from build123d import *

# Parameters (mm, degrees)
SKETCH1_W           = 24
SKETCH1_H           = 24
BOSS_EXTRUDE1_DEPTH = 40
SHELL3_T            = -2
SKETCH3_R           = 11.1
BOSS_EXTRUDE3_DEPTH = 15
SKETCH4_R           = 9.55
CUT_EXTRUDE3_DEPTH  = 12
FILLET4_R           = 0.5
SKETCH2_W           = 20
SKETCH2_H           = 2
BOSS_EXTRUDE5_DEPTH = 40
SKETCH6_W           = 20
SKETCH6_H           = 4
CUT_EXTRUDE4_DEPTH  = 8
SKETCH7_W           = 4
SKETCH7_H           = 18
CUT_EXTRUDE5_DEPTH  = 8
SKETCH8_R           = 2.5
CUT_EXTRUDE6_DEPTH  = 2


with BuildPart() as part:
    # Sketch1 → Boss-Extrude1 (new body)
    with BuildSketch(Plane(origin=(0, 0, 0), x_dir=(1, 0, 0), z_dir=(0, 1, 0))):
        Rectangle(SKETCH1_W, SKETCH1_H)
    extrude(amount=BOSS_EXTRUDE1_DEPTH)

    # Shell3
    shell3_openings = [part.faces().sort_by_distance(p)[0] for p in [
        (0, 40, 0),
        (0, 0, 0),
    ]]
    offset(amount=SHELL3_T, openings=shell3_openings, kind=Kind.INTERSECTION)

    # Sketch3 → Boss-Extrude3 (add)
    with BuildSketch(Plane.XY.offset(12)):
        with Locations((0, 20)):
            Circle(SKETCH3_R)
    extrude(amount=BOSS_EXTRUDE3_DEPTH)

    # Sketch4 → Cut-Extrude3 (cut)
    with BuildSketch(Plane.XY.offset(27)):
        with Locations((0, 20)):
            Circle(SKETCH4_R)
    extrude(amount=-CUT_EXTRUDE3_DEPTH, mode=Mode.SUBTRACT)

    # Fillet4
    fillet4_edges = [part.edges().sort_by_distance(p)[0] for p in [
        (-11.1, 20, 12),
    ]]
    fillet(fillet4_edges, radius=FILLET4_R)

    # Sketch2 → Boss-Extrude5 (add)
    with BuildSketch(Plane(origin=(0, 40, 0), x_dir=(1, 0, 0), z_dir=(0, 1, 0))):
        with Locations((0, 1)):
            Rectangle(SKETCH2_W, SKETCH2_H)
    extrude(amount=-BOSS_EXTRUDE5_DEPTH)

    # Sketch6 → Cut-Extrude4 (cut)
    with BuildSketch(Plane(origin=(11.1, 0, 0), x_dir=(0, 0, -1), z_dir=(1, 0, 0))):
        with Locations((-27, 20)):
            Rectangle(SKETCH6_W, SKETCH6_H)
    extrude(amount=-CUT_EXTRUDE4_DEPTH, mode=Mode.SUBTRACT)

    # Sketch7 → Cut-Extrude5 (cut)
    with BuildSketch(Plane(origin=(0, 8.9, 0), x_dir=(1, 0, 0), z_dir=(0, 1, 0))):
        with Locations((0, -27)):
            Rectangle(SKETCH7_W, SKETCH7_H)
    extrude(amount=CUT_EXTRUDE5_DEPTH, mode=Mode.SUBTRACT)

    # Sketch8 → Cut-Extrude6 (cut)
    with BuildSketch(Plane.XY.offset(12)):
        with Locations((7, 35)):
            Circle(SKETCH8_R)
    cut_extrude6 = extrude(amount=-CUT_EXTRUDE6_DEPTH, mode=Mode.SUBTRACT)

    # Mirror1: Cut-Extrude6 across plane
    add(cut_extrude6.mirror(Plane.ZX.offset(20)), mode=Mode.SUBTRACT)


solid = part.part
Verification items for the finished model (mm, model axes). A direction names the side the tool comes from. Round coordinates to 2 decimals unless told otherwise and drop trailing zeros. Loops run counter-clockwise (first coordinate to the right, second up) from the corner with the lowest first, then second, coordinate; pieces in that order, holes last. Notation, with made-up numbers: (7, -24.75) - (63, -24.75) arc R23 ccw to (63, 8.25) - close; hole circle Ø5 at (51, 89.25). An arc over 180 degrees is marked (long way). Use a Markdown table: item, result. Add a question column.
1. Access from +Z, -Z, +X, -X, +Y, -Y to the whole of each face (thin tool, end or side, straight path). Record for faces 4 (the face through (2, 10, 23)), 5 (the face through (10, 20, -6)), 6 (the face through (10, 20, 17)), 7 (the face through (0, 20, -12)), 8 (the face through (4.41, 11.53, 21.08)).
2. Section check A-A, the plane z = -4. Record the boundary of the cut face in (x, y).
3. Release check for a two-part mould opening along Y. For faces 1 (the face through (0, 20, 15)), 2 (the face through (-5.04, 28.3, 27)), 3 (the face through (-0.2, 0, -0.2)) record: released by +Y, released by -Y, zero draft, split by the parting line, or undercut.
4. Section check D-D, the plane y = 20. Record the boundary of the cut face in (x, z).
5. Gauge pin test, flat ends, axial feed: pin 1 (6 mm diameter, centred on x = 2.5, y = 24.5, fed in from +Z); pin 2 (1.3 mm diameter, centred on y = 10, z = 20.5, fed in from -X); pin 3 (0.5 mm diameter, centred on x = 10.5, z = 22.5, fed in from +Y); pin 4 (12 mm diameter, centred on x = -2.5, y = 16, fed in from +Z). Record the tip position at first contact, or that the pin passes through.
6. Section check B-B, the plane x = 0. Record the boundary of the cut face in (y, z).
7. Thickness scan on probe 1 along Z at (x, y) = (-0.75, 26); probe 2 along Z at (x, y) = (6.75, 31.5); probe 3 along Y at (x, z) = (7, 10.4). Record the ranges inside material, lowest first. Write a range as [from, to].
8. Section check C-C, the plane y = 37. Record the boundary of the cut face in (x, z).
Checks:
| question | item | result |
|---|---|---|
| 1 | face 4 | +Z, -Y |
| 1 | face 5 | +Y, -Y |
| 1 | face 6 | +Z, +X |
| 1 | face 7 | -Z, +X, -X, +Y, -Y |
| 1 | face 8 | +Z |
| 2 | outline | (-12, 0) - (-10, 0) - (-10, 40) - (-12, 40) - close; (10, 0) - (12, 0) - (12, 40) - (10, 40) - close |
| 3 | face 1 | undercut |
| 3 | face 2 | zero draft |
| 3 | face 3 | released by -Y |
| 4 | outline | (-12, -12) - (12, -12) - (12, 12) - (11.6, 12) arc R0.5 cw to (11.1, 12.5) - (11.1, 17) - (9.55, 17) - (9.55, 15) - (-9.55, 15) - (-9.55, 27) - (-11.1, 27) - (-11.1, 12.5) arc R0.5 cw to (-11.6, 12) - (-12, 12) - close; hole (-10, -10) - (10, -10) - (10, -2) - (-10, -2) - close; hole (-10, 0) - (10, 0) - (10, 10) - (-10, 10) - close |
| 5 | pin 1 | stops at z = 15 |
| 5 | pin 2 | stops at x = -5.98 |
| 5 | pin 3 | stops at y = 24.26 |
| 5 | pin 4 | stops at z = 27 |
| 6 | outline | (0, -12) - (40, -12) - (40, -10) - (0, -10) - close; (0, -2) - (40, -2) - (40, 0) - (0, 0) - close; (0, 10) - (40, 10) - (40, 12) - (31.6, 12) arc R0.5 cw to (31.1, 12.5) - (31.1, 27) - (29.55, 27) - (29.55, 15) - (10.45, 15) - (10.45, 18) - (8.9, 18) - (8.9, 12.5) arc R0.5 cw to (8.4, 12) - (0, 12) - close |
| 7 | probe 1 | z = [-12, -10], [-2, 0], [10, 15] |
| 7 | probe 2 | z = [-12, -10], [-2, 0], [10, 12] |
| 7 | probe 3 | y = [0, 2.5], [7.5, 32.5], [37.5, 40] |
| 8 | outline | (-12, -12) - (12, -12) - (12, 12) - (8.5, 12) - (8.5, 10) - (10, 10) - (10, 0) - (-10, 0) - (-10, 10) - (5.5, 10) - (5.5, 12) - (-12, 12) - close; hole (-10, -10) - (10, -10) - (10, -2) - (-10, -2) - close |
